Work out the finished part from the listing and answer in its coordinate system (mm). A direction names the side the tool comes from. Give positions to 0.01 mm unless a question says otherwise; leave off trailing zeros. Order: outer loops, then holes, each group sorted by start corner. A loop starts at its lowest first (then second) coordinate and runs counter-clockwise, first axis right, second up. Notation, with made-up numbers: (79, 54) - (87, 54) arc R33 ccw to (87, 85) - close; hole circle Ø8 at (44.5, 12). An arc over 180 degrees is marked (long way). Put each result on its own line as item: value.
```python
from build123d import *

# Parameters (mm, degrees)
SKETCH1_R           = 75
BOSS_EXTRUDE1_DEPTH = 1187
SKETCH3_W           = 824.711862224
SKETCH3_H           = 100
BOSS_EXTRUDE2_DEPTH = 874


with BuildPart() as part:
    # Sketch1 → Boss-Extrude1 (new body)
    with BuildSketch(Plane.XY):
        with Locations(Location((0, 0, 0), (0, 0, 180))):
            Circle(SKETCH1_R)
    extrude(amount=BOSS_EXTRUDE1_DEPTH)

    # Sketch3 → Boss-Extrude2 (add)
    with BuildSketch(Plane(origin=(10, 0, 0), x_dir=(0, 0, -1), z_dir=(1, 0, 0))):
        with Locations((-603.421893573, -6.041666237)):
            Rectangle(SKETCH3_W, SKETCH3_H)
    extrude(amount=BOSS_EXTRUDE2_DEPTH)


solid = part.part
```
(1) Given pin 1 (6 mm diameter, centred on y = -50, z = 364, fed in from -X); pin 2 (12 mm diameter, centred on x = 739, z = 508, fed in from -Y); pin 3 (1.5 mm diameter, centred on x = 173, z = 757.5, fed in from +Y), each flat-ended and moving along its own axis, determine where each tip first touches the part or whether it passes through.
Geometry check:
pin 1: stops at x = -58.45
pin 2: stops at y = -56.04
pin 3: stops at y = 43.96
(2) Section A-A, the plane y = 0 is taken. Write down the section's boundary in (x, z), then the cut area to 3 significant figures.
Geometry check:
outline: (-75, 0) - (75, 0) - (75, 191.07) - (884, 191.07) - (884, 1015.78) - (75, 1015.78) - (75, 1187) - (-75, 1187) - close
area: 845,000 mm²
(3) A tool of negligible diameter and unlimited length cuts with its end or side. For faces 1 (the face through (467, 43.958, 609)), 2 (the face through (1, -1, 1187)), 3 (the face through (461, -56.042, 609)), from which of +Z, -Z, +X, -X, +Y, -Y can it reach the whole face along a straight path? Write none if from no direction.
Geometry check:
face 1: +Z, -Z, +X, +Y
face 2: +Z, +X, -X, +Y, -Y
face 3: +Z, -Z, +X, -Y
(4) Section C-C, the plane x = 446.5 is taken. Write down the section's boundary in (y, z), then the cut area to 3 significant figures.
Geometry check:
outline: (-56.04, 191.07) - (43.96, 191.07) - (43.96, 1015.78) - (-56.04, 1015.78) - close
area: 82,500 mm²
(5) Straight lines are drawn through the part: line 1 (Y direction, x = 759.5, z = 660.5); line 2 (Z direction, x = 516, y = 33); line 3 (X direction, y = -45, z = 94). For each, find the intervals that lie inside material, in ascending order.
Geometry check:
line 1: y = -56.04 to 43.96
line 2: z = 191.07 to 1015.78
line 3: x = -60 to 60
(6) Section B-B, the plane z = 517 is taken. Write down the section's boundary in (x, y), then the cut area to 3 significant figures.
Geometry check:
outline: (49.84, -56.04) - (884, -56.04) - (884, 43.96) - (60.77, 43.96) arc R75 ccw (long way) to start
area: 99,200 mm²
